The drawing under review shows one solid part. Ordinate dimensions are in mm from its lowest x, y, z. Give positions to 0.01 mm unless a question says otherwise; leave off trailing zeros. Write each loop counter-clockwise with the first axis right and the second up, starting at its lowest first coordinate (ties: lowest second). Pieces come first, ordered by that corner, then holes. Notation, with made-up numbers: (4, 12) -> (27, 12) arc R21 cw to (27, 22) -> close; hole circle Ø9 at (29.25, 86). An arc over 180 degrees is marked (long way). Write item = value, one per line.
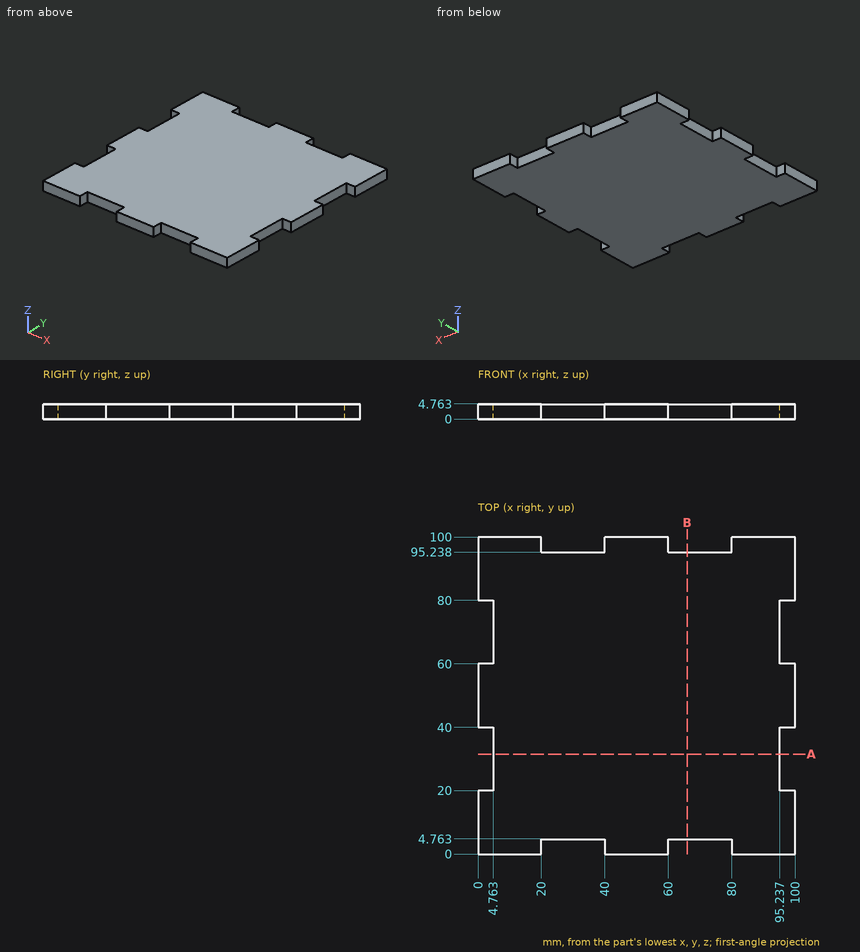
(1) Take a section at A-A (y = 31.5). Write out the cut boundary in (x, z).
Answers below:
outline = (4.76, 0) -> (95.24, 0) -> (95.24, 4.76) -> (4.76, 4.76) -> close
(2) For pin 1 (1 mm diameter, centred on x = 67.5, z = 2, fed in from +Y); pin 2 (2.5 mm diameter, centred on y = 31.5, z = 1.5, fed in from -X); pin 3 (1.4 mm diameter, centred on x = 74.5, z = 2.5, fed in from -Y), all flat-tipped, find the tip position at first contact; note any pin that passes through.
Answers below:
pin_1 = 95.24
pin_2 = 4.76
pin_3 = 4.76
(3) To check wall thickness, follow probe 1 along Y at (x, z) = (26.5, 1.4). State the ranges of the line that lie inside material, in increasing order.
Answers below:
probe_1 = 4.76 to 95.24
